Verification items for the finished model (mm, model axes). Face numbers are marked on the shaded views. A direction names the side the tool comes from. Coordinates: 2 decimals unless noted, no trailing zeros. Order: outer loops, then holes, each group sorted by start corner. A loop starts at its lowest first (then second) coordinate and runs counter-clockwise, first axis right, second up. Notation, with made-up numbers: (21, 19.25) -> (35, 19.25) arc R8 cw to (35, 31.25) -> close; hole circle Ø11 at (48.25, 21.5). An arc over 180 degrees is marked (long way). Write item = value, one per line. Start each with the question number.
1. Cross-section at C-C on z = 0. Record the cut outline in (x, y).
2. Cross-section at D-D on x = 8. Record the cut outline in (y, z).
3. Release check for a two-part mould opening along Z. For the marked faces 5, 6, 7 and 8 record: +Z half, -Z half, draft (parallel to the pull), parting line (faces both ways), or undercut.
4. Thickness scan on line 1 along X through (y, z) = (-1, -0.25); line 2 along X through (y, z) = (2.5, 4.75); line 3 along Z through (x, y) = (0.5, 2.5). Record the ranges inside material, lowest first. Write a range as from..to.
5. Set-up check for the marked faces 1, 2, 3 and 4: record each of +Z, -Z, +X, -X, +Y, -Y from which the full face is reachable in a straight line by a thin tool's end or side.
6. Cross-section at B-B on y = 0. Record the cut outline in (x, z).
7. Go/stop test with a flat-tipped pin: P1, Ø2, axis at y = 0, z = 6, coming from the +X side. Record where the tip stops, or that it passes through.
8. Cross-section at A-A on z = -7. Record the cut outline in (x, y), plus the area to 3 significant figures.
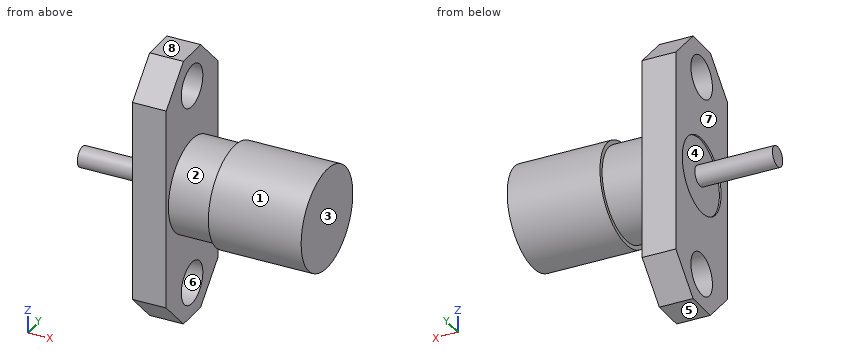
from build123d import *

# Parameters (mm, degrees)
SKETCH_1_R          = 1.25
EXTRUDE_1_DEPTH     = 2
SKETCH_2_R          = 2.25
CUT_EXTRUDE_1_DEPTH = 0.1
SKETCH_6_R          = 0.6
EXTRUDE_2_DEPTH     = 4.6
SKETCH_7_R          = 3
EXTRUDE_3_DEPTH     = 8
SKETCH_8_W          = 2.5
SKETCH_8_H          = 0.25


with BuildPart() as part:
    # Эскиз1 → Бобышка-Вытянуть1 (new body)
    with BuildSketch(Plane(origin=(0, 0, 0), x_dir=(0, 0, -1), z_dir=(1, 0, 0))):
        Polygon((-6, 3), (-8, 1), (-8, -1), (-6, -3), (6, -3), (8, -1), (8, 1), (6, 3), align=None)
        with Locations((-6, 0)):
            Circle(SKETCH_1_R, mode=Mode.SUBTRACT)
        with Locations((6, 0)):
            Circle(SKETCH_1_R, mode=Mode.SUBTRACT)
    extrude(amount=EXTRUDE_1_DEPTH)

    # Эскиз2 → Вырез-Вытянуть1 (cut)
    with BuildSketch(Plane.ZY):
        Circle(SKETCH_2_R)
    extrude(amount=-CUT_EXTRUDE_1_DEPTH, mode=Mode.SUBTRACT)

    # Эскиз6 → Бобышка-Вытянуть2 (add)
    with BuildSketch(Plane.ZY.offset(-0.1)):
        Circle(SKETCH_6_R)
    extrude(amount=EXTRUDE_2_DEPTH)

    # Эскиз7 → Бобышка-Вытянуть3 (add)
    with BuildSketch(Plane(origin=(2, 0, 0), x_dir=(0, 0, -1), z_dir=(1, 0, 0))):
        with Locations(Location((0, 0, 0), (0, 0, 270))):
            Circle(SKETCH_7_R)
    extrude(amount=EXTRUDE_3_DEPTH)

    # Эскиз8 → Вырез-Повернуть1 (revolve, cut)
    with BuildSketch(Plane.XY, mode=Mode.PRIVATE) as cut_revolve_1_sk:
        with Locations((3.25, 2.875)):
            Rectangle(SKETCH_8_W, SKETCH_8_H)
    revolve(cut_revolve_1_sk.sketch.rotate(Axis((-1000, 0, 0), (1, 0, 0)), 90), axis=Axis((-1000, 0, 0), (1, 0, 0)), mode=Mode.SUBTRACT)


solid = part.part
Worked out:
q1.outline = (-4.5, -0.6) -> (0.1, -0.6) -> (0.1, -2.25) -> (0, -2.25) -> (0, -3) -> (2, -3) -> (2, -2.75) -> (4.5, -2.75) -> (4.5, -3) -> (10, -3) -> (10, 3) -> (4.5, 3) -> (4.5, 2.75) -> (2, 2.75) -> (2, 3) -> (0, 3) -> (0, 2.25) -> (0.1, 2.25) -> (0.1, 0.6) -> (-4.5, 0.6) -> close
q2.outline = circle Ø6 at (0, 0)
q3.face_5 = -Z half
q3.face_6 = undercut
q3.face_7 = draft
q3.face_8 = +Z half
q4.line_1 = 0.1..10
q4.line_2 = 0..2
q4.line_3 = -6.5..6.5
q5.face_1 = +X
q5.face_2 = none
q5.face_3 = +Z, -Z, +X, +Y, -Y
q5.face_4 = -X
q6.outline = (-4.5, -0.6) -> (0.1, -0.6) -> (0.1, -2.25) -> (0, -2.25) -> (0, -4.75) -> (2, -4.75) -> (2, -2.75) -> (4.5, -2.75) -> (4.5, -3) -> (10, -3) -> (10, 3) -> (4.5, 3) -> (4.5, 2.75) -> (2, 2.75) -> (2, 4.75) -> (0, 4.75) -> (0, 2.25) -> (0.1, 2.25) -> (0.1, 0.6) -> (-4.5, 0.6) -> close; (0, -8) -> (2, -8) -> (2, -7.25) -> (0, -7.25) -> close; (0, 7.25) -> (2, 7.25) -> (2, 8) -> (0, 8) -> close
q7.P1 = through
q8.outline = (0, -2) -> (2, -2) -> (2, -0.75) -> (0, -0.75) -> close; (0, 0.75) -> (2, 0.75) -> (2, 2) -> (0, 2) -> close
q8.area = 5.00 mm²
